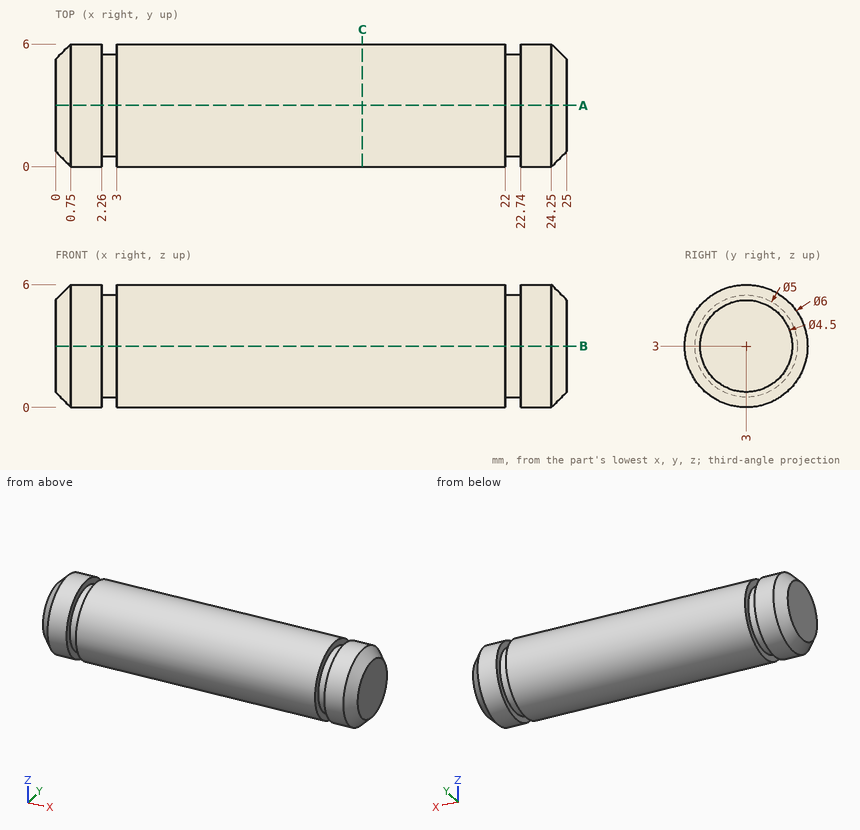
For this review, use the dimensioned drawing (mm, ordinates from the lowest corner) and the shaded views. Round coordinates to 2 decimals unless told otherwise and drop trailing zeros. Write each loop counter-clockwise with the first axis right and the second up, starting at its lowest first coordinate (ties: lowest second). Pieces come first, ordered by that corner, then holes. Notation, with made-up numbers: (-9.5, 7) -> (6.5, 7) arc R34 ccw to (6.5, 45) -> close; hole circle Ø6 at (32.25, 19.5). An arc over 180 degrees is marked (long way). Use one line per item in the form item = value.
Q1. To check wall thickness, follow probe 1 along X at (y, z) = (3.2, 0.45); probe 2 along Y at (x, z) = (20, 5.2); probe 3 along Z at (x, y) = (16.25, 1). State the ranges of each line that lie inside material, in increasing order. Write a range as from..to.
Resolved:
probe_1 = 0.31..2.26, 3..22, 22.74..24.69
probe_2 = 0.96..5.04
probe_3 = 0.76..5.24
Q2. Clearance check with flat-ended pins moving along their axes: pin 1 Ø1 at (x, y) = (9, 5) entering from +Z; pin 2 Ø1 at (x, y) = (8.5, 1.5) entering from -Z. State where each tip first meets the part, or that it passes through.
Resolved:
pin_1 = 5.6
pin_2 = 0.17
Q3. Consider section A-A (y = 3). State the section outline as (x, z) points.
Resolved:
outline = (0, 0.75) -> (0.75, 0) -> (2.26, 0) -> (2.26, 0.5) -> (3, 0.5) -> (3, 0) -> (22, 0) -> (22, 0.5) -> (22.74, 0.5) -> (22.74, 0) -> (24.25, 0) -> (25, 0.75) -> (25, 5.25) -> (24.25, 6) -> (22.74, 6) -> (22.74, 5.5) -> (22, 5.5) -> (22, 6) -> (3, 6) -> (3, 5.5) -> (2.26, 5.5) -> (2.26, 6) -> (0.75, 6) -> (0, 5.25) -> close
Q4. Consider section C-C (x = 15). State the section outline as (y, z) points.
Resolved:
outline = circle Ø6 at (3, 3)
